Check sheet for the modelled part. Datum: model origin and axes. Units: mm. Face numbers are marked on the shaded views. A direction names the side the tool comes from. Coordinates: 2 decimals unless noted, no trailing zeros. Loops run counter-clockwise (first coordinate to the right, second up) from the corner with the lowest first, then second, coordinate; pieces in that order, holes last. Notation, with made-up numbers: (-35.75, 27.5) - (-14.75, 27.5) arc R20 ccw to (-14.75, 63.5) - close; hole circle Ø3 at (45.5, 4.5). An arc over 180 degrees is marked (long way). Write each question's results on one line, items separated by ' | '. Start each with the question number.
1. Tool access check on the marked faces 4, 5, 6 and 7. Record the directions out of +Z, -Z, +X, -X, +Y, -Y that give a thin tool (end or side, any length) a straight path to the whole face; none if there is none.
2. Cross-section at A-A (y = -8.5). Give the number of separate pieces and of enclosed holes in the cut face, and give its area (3 significant figures).
3. Cross-section at D-D (x = 0). Record the cut outline in (y, z).
4. Cross-section at C-C (z = 6). Record the cut outline in (x, y), and give its area (3 significant figures).
5. Thickness scan on line 1 (Z direction, x = -9, y = -6.5); line 2 (X direction, y = -1.25, z = -9.5); line 3 (X direction, y = 4.75, z = 2.5). Record the ranges inside material, lowest first. Write a range as [from, to].
6. Cross-section at B-B (x = 9.5). Record the cut outline in (y, z), and give its area (3 significant figures).
7. Gauge pin test, flat ends, axial feed: P1, Ø1, axis at y = -11, z = 6, coming from the +X side; P2, Ø5, axis at x = -6.5, y = 6.5, coming from the +Z side; P3, Ø6.5, axis at x = -7, y = -3.5, coming from the -Z side; P4, Ø6.5, axis at y = -1, z = 8, coming from the -X side. Record the tip position at first contact, or that the pin passes through.
8. Draft check along X on the marked faces 1, 2 and 3. Enter one of: released by +X, released by -X, zero draft, split by the parting line, or undercut.
```python
from build123d import *

# Parameters (mm, degrees)
F0_R     = 13
F1_DEPTH = 10
F2_R     = 2.5
F3_DEPTH = 14
F4_SIZE  = 0.5


with BuildPart() as f1:
    # F0 (on Front) → F1 (new body, symmetric)
    with BuildSketch(Plane.XZ):
        Circle(F0_R)
        with BuildLine():
            ThreePointArc((-2.738095, -11.169281), (-8.131728, -8.131728), (-11.169281, -2.738095))
            ThreePointArc((-11.169281, -2.738095), (-10.984835, -1.882787), (-10.198039, -1.5))
            Line((-10.198039, -1.5), (-4.330127, -1.5))
            ThreePointArc((-4.330127, -1.5), (-3.830127, -1.633975), (-3.464102, -2))
            ThreePointArc((-3.464102, -2), (-2.828427, -2.828427), (-2, -3.464102))
            ThreePointArc((-2, -3.464102), (-1.633975, -3.830127), (-1.5, -4.330127))
            Line((-1.5, -4.330127), (-1.5, -10.198039))
            ThreePointArc((-1.5, -10.198039), (-1.882787, -10.984835), (-2.738095, -11.169281))
        make_face(mode=Mode.SUBTRACT)
        with BuildLine():
            Line((1.5, -10.198039), (1.5, -4.330127))
            ThreePointArc((1.5, -4.330127), (1.633975, -3.830127), (2, -3.464102))
            ThreePointArc((2, -3.464102), (2.828427, -2.828427), (3.464102, -2))
            ThreePointArc((3.464102, -2), (3.830127, -1.633975), (4.330127, -1.5))
            Line((4.330127, -1.5), (10.198039, -1.5))
            ThreePointArc((10.198039, -1.5), (10.984835, -1.882787), (11.169281, -2.738095))
            ThreePointArc((11.169281, -2.738095), (8.131728, -8.131728), (2.738095, -11.169281))
            ThreePointArc((2.738095, -11.169281), (1.882787, -10.984835), (1.5, -10.198039))
        make_face(mode=Mode.SUBTRACT)
        with BuildLine():
            ThreePointArc((-1.5, 4.330127), (-1.633975, 3.830127), (-2, 3.464102))
            ThreePointArc((-2, 3.464102), (-2.828427, 2.828427), (-3.464102, 2))
            ThreePointArc((-3.464102, 2), (-3.830127, 1.633975), (-4.330127, 1.5))
            Line((-4.330127, 1.5), (-10.198039, 1.5))
            ThreePointArc((-10.198039, 1.5), (-10.984835, 1.882787), (-11.169281, 2.738095))
            ThreePointArc((-11.169281, 2.738095), (-8.131728, 8.131728), (-2.738095, 11.169281))
            ThreePointArc((-2.738095, 11.169281), (-1.882787, 10.984835), (-1.5, 10.198039))
            Line((-1.5, 10.198039), (-1.5, 4.330127))
        make_face(mode=Mode.SUBTRACT)
        with BuildLine():
            Line((1.5, 4.330127), (1.5, 10.198039))
            ThreePointArc((1.5, 10.198039), (1.882787, 10.984835), (2.738095, 11.169281))
            ThreePointArc((2.738095, 11.169281), (8.131728, 8.131728), (11.169281, 2.738095))
            ThreePointArc((11.169281, 2.738095), (10.984835, 1.882787), (10.198039, 1.5))
            Line((10.198039, 1.5), (4.330127, 1.5))
            ThreePointArc((4.330127, 1.5), (3.830127, 1.633975), (3.464102, 2))
            ThreePointArc((3.464102, 2), (2.828427, 2.828427), (2, 3.464102))
            ThreePointArc((2, 3.464102), (1.633975, 3.830127), (1.5, 4.330127))
        make_face(mode=Mode.SUBTRACT)
    extrude(amount=F1_DEPTH, both=True)

    # F2 (on Front) → F3 (join, symmetric)
    with BuildSketch(Plane.XZ):
        Circle(F2_R)
    extrude(amount=F3_DEPTH, both=True)

    # F4
    f4_edges = [f1.edges().sort_by_distance(p)[0] for p in [
        (-2.5, -14, 0),
        (-2.5, 14, 0),
    ]]
    chamfer(f4_edges, length=F4_SIZE)


solid = f1.part
```
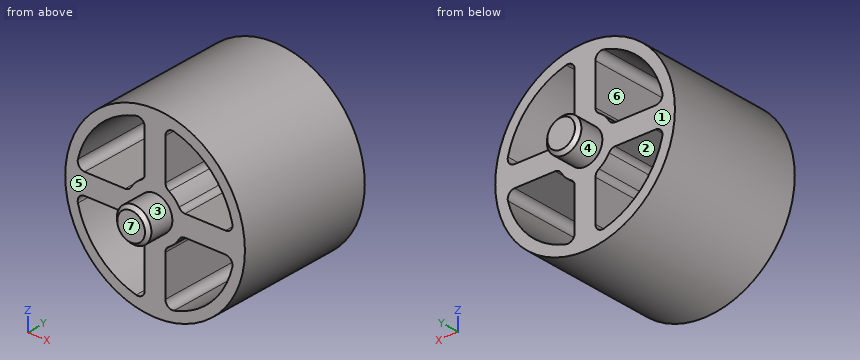
Established:
1) face 4: +Y | face 5: -Y | face 6: +Y, -Y | face 7: +Z, -Z, +X, -X, -Y
2) separate pieces: 1 | enclosed holes: 4 | area: 260 mm^2
3) outline: (-14, -2) - (-13.5, -2.5) - (-10, -2.5) - (-10, -13) - (10, -13) - (10, -2.5) - (13.5, -2.5) - (14, -2) - (14, 2) - (13.5, 2.5) - (10, 2.5) - (10, 13) - (-10, 13) - (-10, 2.5) - (-13.5, 2.5) - (-14, 2) - close
4) outline: (-11.53, -10) - (-9.81, -10) - (-9.81, 10) - (-11.53, 10) - close; (-1.5, -10) - (1.5, -10) - (1.5, 10) - (-1.5, 10) - close; (9.81, -10) - (11.53, -10) - (11.53, 10) - (9.81, 10) - close | area: 129 mm^2
5) line 1: [-9.38, -7.16], [-1.5, 1.5], [7.16, 9.38] | line 2: [-8.87, -6.48], [-1.5, 1.5], [6.48, 8.87] | line 3: [-12.76, -11.2], [-3.12, 3.12], [11.2, 12.76]
6) outline: (-10, -8.87) - (10, -8.87) - (10, -6.48) - (-10, -6.48) - close; (-10, -1.5) - (10, -1.5) - (10, 1.5) - (-10, 1.5) - close; (-10, 6.48) - (10, 6.48) - (10, 8.87) - (-10, 8.87) - close | area: 156 mm^2
7) P1: through | P2: z = 12.37 | P3: z = -12.45 | P4: x = -12.1
8) face 1: zero draft | face 2: undercut | face 3: split by the parting line
